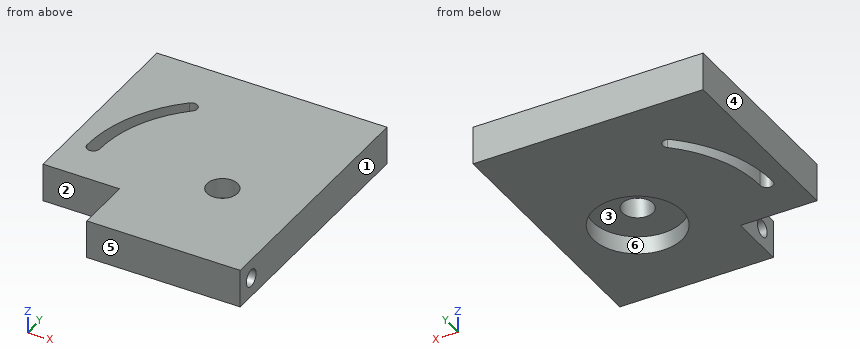
```python
from build123d import *

# Parameters (mm, degrees)
SKETCH_1_W                   = 90.133378614
SKETCH_1_H                   = 100
EXTRUDE_1_DEPTH              = 15
HOLE_WIZARD_M101_D           = 12
HOLE_WIZARD_M101_CBORE_D     = 35
HOLE_WIZARD_M101_CBORE_DEPTH = 7
SKETCH_10_W                  = 15
SKETCH_10_H                  = 22.389140256
CUT_EXTRUDE_3_DEPTH          = 30
SKETCH_12_R                  = 3.35
CUT_EXTRUDE_4_DEPTH          = 10
CUT_EXTRUDE_START            = -10
SKETCH_14_R                  = 3.35
CUT_EXTRUDE_5_DEPTH          = 10
CUT_EXTRUDE_6_DEPTH          = 87.261365764


with BuildPart() as part:
    # Эскиз1 → Бобышка-Вытянуть1 (new body)
    with BuildSketch(Plane.XY.offset(15)):
        with Locations((-15.066689307, 10)):
            Rectangle(SKETCH_1_W, SKETCH_1_H)
    extrude(amount=-EXTRUDE_1_DEPTH)

    # Цековка для  болта с шестигранной головкой M101 (through all)
    with Locations(Plane(origin=(0, 0, 0), x_dir=(-1, 0, 0), z_dir=(0, 0, -1))):
        with Locations((0, 0)):
            CounterBoreHole(HOLE_WIZARD_M101_D / 2, HOLE_WIZARD_M101_CBORE_D / 2, HOLE_WIZARD_M101_CBORE_DEPTH)

    # Эскиз10 → Вырез-Вытянуть3 (cut)
    with BuildSketch(Plane.ZY.offset(60.133378614)):
        with Locations((7.5, -28.805429872)):
            Rectangle(SKETCH_10_W, SKETCH_10_H)
    extrude(amount=-CUT_EXTRUDE_3_DEPTH, mode=Mode.SUBTRACT)

    # Эскиз12 → Вырез-Вытянуть4 (cut)
    with BuildSketch(Plane.ZY.offset(30.133378614)):
        with Locations(Location((7.5, -32.5, 0), (0, 0, 270))):
            Circle(SKETCH_12_R)
    extrude(amount=-CUT_EXTRUDE_4_DEPTH, mode=Mode.SUBTRACT)

    # Эскиз14 → Вырез-Вытянуть5 (cut)
    with BuildSketch(Plane(origin=(30, 0, 0), x_dir=(0, 0, -1), z_dir=(1, 0, 0)).offset(CUT_EXTRUDE_START)):
        with Locations(Location((-7.5, -32.5, 0), (0, 0, 270))):
            Circle(SKETCH_14_R)
    extrude(amount=CUT_EXTRUDE_5_DEPTH, mode=Mode.SUBTRACT)

    # Эскиз18 → Вырез-Вытянуть6 (cut, through all)
    with BuildSketch(Plane.XY.offset(15)):
        with BuildLine():
            ThreePointArc((-35.524835884, 39.336218188), (-48.437001879, 21.522287864), (-53.003320895, 0))
            ThreePointArc((-53.003320895, 0), (-50.503320895, -2.5), (-48.003320895, 0))
            ThreePointArc((-48.003320895, 0), (-43.867759701, 19.492010563), (-32.173646253, 35.625486717))
            ThreePointArc((-32.173646253, 35.625486717), (-31.993875333, 39.156447268), (-35.524835884, 39.336218188))
        make_face()
    extrude(amount=-CUT_EXTRUDE_6_DEPTH, mode=Mode.SUBTRACT)


solid = part.part
```
CAD build for the part. Positions are in the model's coordinates, mm. Face numbers are marked on the shaded views. A direction names the side the tool comes from. Give positions to 0.01 mm unless a question says otherwise; leave off trailing zeros. Loops run counter-clockwise (first coordinate to the right, second up) from the corner with the lowest first, then second, coordinate; pieces in that order, holes last. Notation, with made-up numbers: (85, -7.5) - (106, -7.5) arc R22 cw to (106, -0.5) - close; hole circle Ø1 at (14.25, 32.5). An arc over 180 degrees is marked (long way). Put each result on its own line as item: value.
Q1. Slice it at C-C (z = 13.75). Give the cut face in (x, y).
Filled in:
outline: (-60.13, -17.61) - (-30.13, -17.61) - (-30.13, -40) - (30, -40) - (30, 60) - (-60.13, 60) - close; hole (-53, 0) arc R2.5 ccw to (-48, 0) arc R48 cw to (-32.17, 35.63) arc R2.5 ccw to (-35.52, 39.34) arc R53 ccw to start; hole circle Ø12 at (0, 0)
Q2. Tool access for the marked faces 1, 2 and 3: list every direction of +Z, -Z, +X, -X, +Y, -Y with a clear straight run to the whole face (end or side of a thin tool).
Filled in:
face 1: +Z, -Z, +X, +Y, -Y
face 2: +Z, -Z, -X, -Y
face 3: -Z
Q3. Probe line 1 along X through (y, z) = (8, 1); line 2 along Y through (x, z) = (0, 13.25); line 3 along Y through (x, z) = (0, 4.75). List the from-to ranges inside material, lowest first.
Filled in:
line 1: x = -60.13 to -52.4, -47.33 to -15.56, 15.56 to 30
line 2: y = -40 to -6, 6 to 60
line 3: y = -40 to -17.5, 17.5 to 60
Q4. Slice it at D-D (y = -32.5). Give the cut face in (x, z), plus the area to 3 significant figures.
Filled in:
outline: (-30.13, 0) - (30, 0) - (30, 4.15) - (20, 4.15) - (20, 10.85) - (30, 10.85) - (30, 15) - (-30.13, 15) - (-30.13, 10.85) - (-20.13, 10.85) - (-20.13, 4.15) - (-30.13, 4.15) - close
area: 768 mm²
Q5. Slice it at A-A (x = 0). Give the cut face in (y, z), plus the area to 3 significant figures.
Filled in:
outline: (-40, 0) - (-17.5, 0) - (-17.5, 7) - (-6, 7) - (-6, 15) - (-40, 15) - close; (6, 7) - (17.5, 7) - (17.5, 0) - (60, 0) - (60, 15) - (6, 15) - close
area: 1,160 mm²
Q6. Slice it at B-B (y = 26). Give the cut face in (x, z), plus the area to 3 significant figures.
Filled in:
outline: (-60.13, 0) - (-46.19, 0) - (-46.19, 15) - (-60.13, 15) - close; (-40.35, 0) - (30, 0) - (30, 15) - (-40.35, 15) - close
area: 1,260 mm²
Q7. Mould opens along X. For the marked faces 4, 5 and 6 say: pulls with the +X half, pulls with the -X half, needs draft (parallel to the pull), parting line crosses it, or undercut.
Filled in:
face 4: pulls with the -X half
face 5: needs draft
face 6: undercut
Q8. Flat gauge pins, fed straight in: pin 1 (1 mm diameter, centred on x = -19, y = -15.5, fed in from -Z); pin 2 (7.5 mm diameter, centred on y = -29.5, z = 10, fed in from -X). Where does each tip first touch, or does it go through?
Filled in:
pin 1: stops at z = 0
pin 2: stops at x = -30.13
